Verification items for this drawing (mm, ordinates from the low corner). A direction names the side the tool comes from. Coordinates: 2 decimals unless noted, no trailing zeros. Write each loop counter-clockwise with the first axis right and the second up, starting at its lowest first coordinate (ties: lowest second). Pieces come first, ordered by that corner, then holes. Notation, with made-up numbers: M 35.5,70.5 L 76.5,70.5 A20 cw 76.5,102.5 Z; hole C -5,53.25 d6. An arc over 180 degrees is marked long. Answer as CSV lines item,"result". Start each with the question number.
1) Access from +Z, -Z, +X, -X, +Y, -Y to the whole of each face (thin tool, end or side, straight path). Record for the marked faces 1, 2 and 3.
2) Section check A-A (x = 38.5). Record the cut outline in (y, z).
3) Material ranges on L1, parallel to X at y = 47, z = 76; L2, parallel to X at y = 7, z = 19; L3, parallel to Y at x = 9, z = 40, recorded low to high. Write a range as [from, to].
4) Draft check along Z on the marked faces 4, 5, 6 and 7. Enter one of: +Z half, -Z half, draft (parallel to the pull), parting line (faces both ways), or undercut.
5) Section check B-B (x = 17.5). Record the cut outline in (y, z), and give its area (3 significant figures).
6) Go/stop test with flat-tipped pins: pin 1 Ø1 at (x, y) = (28, 20.5) entering from -Z (1 decimal); pin 2 Ø12 at (x, z) = (16, 29.5) entering from +Y; pin 3 Ø5 at (x, z) = (5, 71.5) entering from -Y. Record where each tip stops, or that it passes through.
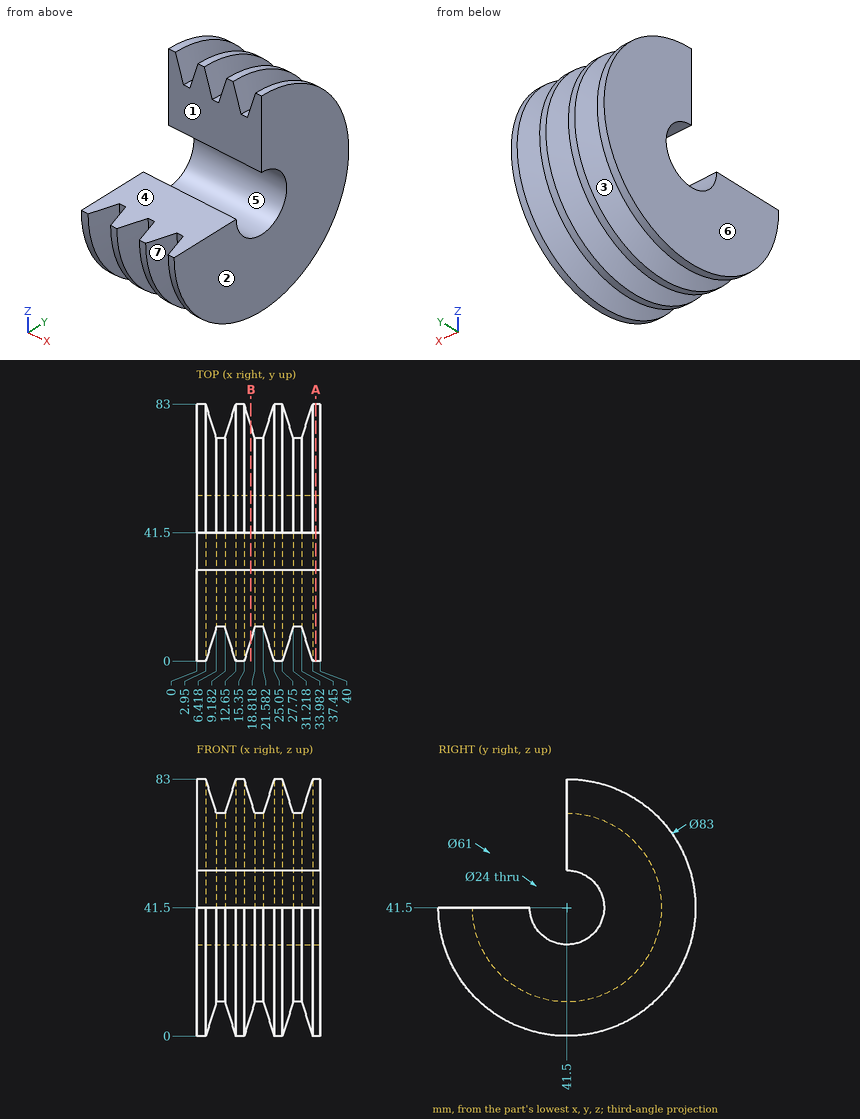
Results found:
1,face 1,"+Z, +X, -X, -Y"
1,face 2,"+Z, -Z, +X, +Y, -Y"
1,face 3,"none"
2,outline,"M 0,41.5 A41.5 ccw long 41.5,83 L 41.5,53.5 A12 cw long 29.5,41.5 Z"
3,L1,"x = [0, 5.02], [10.58, 17.42], [22.98, 29.82], [35.38, 40]"
3,L2,"x = [0, 3.05], [12.55, 15.45], [24.95, 27.85], [37.35, 40]"
3,L3,"y = [11.04, 29.59], [53.41, 71.96]"
4,face 4,"+Z half"
4,face 5,"undercut"
4,face 6,"draft"
4,face 7,"parting line"
5,outline,"M 6.82,41.5 A34.68 ccw long 41.5,76.18 L 41.5,53.5 A12 cw long 29.5,41.5 Z"
5,area,"2,490 mm2"
6,pin 1,"stops at z = 5.5"
6,pin 2,"stops at y = 82.56"
6,pin 3,"stops at y = 41.5"
